Drawing for the job (mm, zero at the part's lowest x, y, z). A direction names the side the tool comes from. Give positions to 0.01 mm unless a question says otherwise; leave off trailing zeros. Write each loop counter-clockwise with the first axis right and the second up, starting at its lowest first coordinate (ties: lowest second). Pieces come first, ordered by that corner, then holes. Notation, with made-up numbers: M -1.5,3 L 40.5,3 A27 cw 40.5,25 Z; hole C -33,39.25 d6. An arc over 180 degrees is marked long. Use CSV: the item, a comma, the result in double quotes. Start each with the question number.
1. Band-saw the part on D-D, the plane z = 17. List the corners of the cut face in (x, y), then the cut area to 3 significant figures.
2. Band-saw the part on A-A, the plane x = 36.5. List the corners of the cut face in (y, z), then the cut area to 3 significant figures.
3. 3-axis set-ups, long thin cutter, end or side, ignore diameter. For the marked faces 1, 2, 3 and 4: which of +Z, -Z, +X, -X, +Y, -Y reach the whole face in a straight line?
4. Drop flat-ended pins along their axis: pin 1 Ø4.5 at (x, y) = (14, 8) entering from +Z; pin 2 Ø6 at (x, y) = (20.5, 43.5) entering from +Z; pin 3 Ø3 at (y, z) = (5, 30) entering from +X. Give the stop position or say it passes through.
5. Drill centre lines: line 1 along Y through (x, z) = (60, 21); line 2 along Z through (x, y) = (67, 20); line 3 along Y through (x, z) = (60, 26). Where is each one in solid material? Low to high. Write a range as from..to.
6. Mould opens along X. For the marked faces 5, 6 and 7 say: pulls with the +X half, pulls with the -X half, needs draft (parallel to the pull), parting line crosses it, or undercut.
7. Band-saw the part on B-B, the plane z = 8. List the corners of the cut face in (x, y).
8. Band-saw the part on C-C, the plane y = 53. List the corners of the cut face in (x, z).
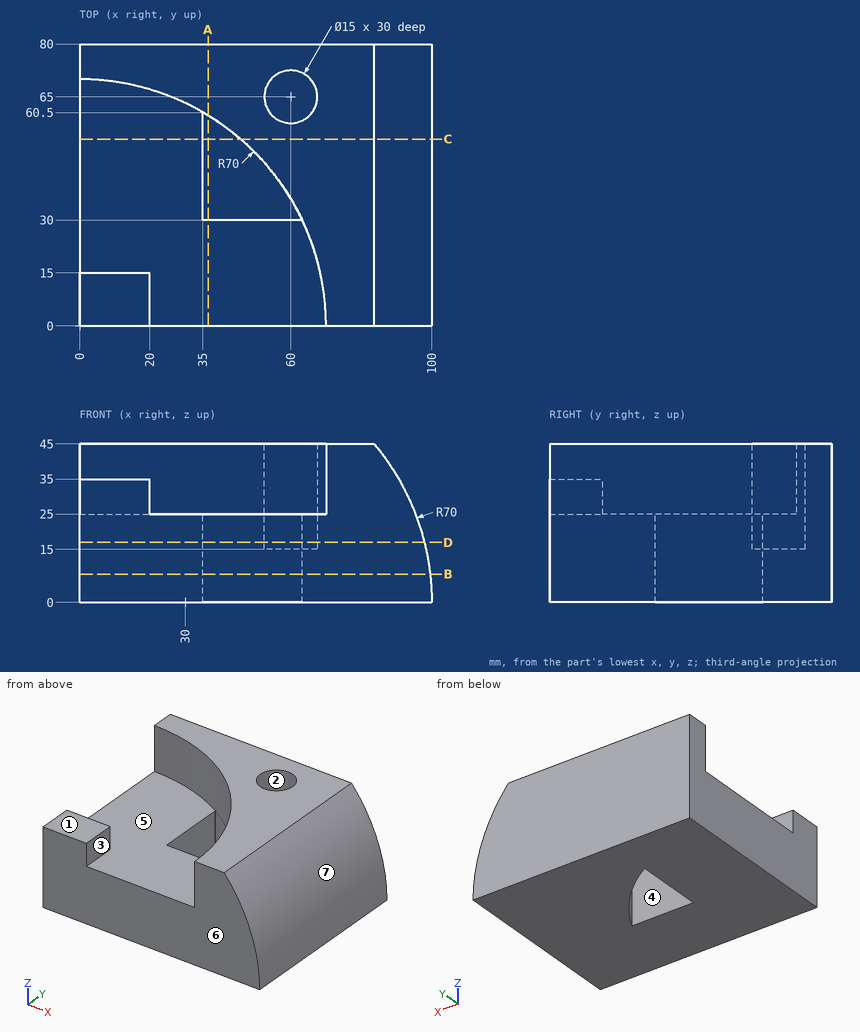
Output:
1,outline,"M 0,0 L 97.9,0 L 97.9,80 L 0,80 Z; hole M 35,30 L 63.25,30 A70 ccw 35.21,60.5 L 35,60.5 Z; hole C 60,65 d15"
1,area,"7,130 mm²"
2,outline,"M 0,0 L 30,0 L 30,25 L 0,25 Z; M 59.73,0 L 80,0 L 80,45 L 59.73,45 Z"
2,area,"1,660 mm²"
3,face 1,"+Z, -X, -Y"
3,face 2,"+Z"
3,face 3,"+Z, -Y"
3,face 4,"+Z, -Z"
4,pin 1,"stops at z = 35"
4,pin 2,"stops at z = 25"
4,pin 3,"stops at x = 93.94"
5,line 1,"y = 0..30, 36.06..57.5, 72.5..80"
5,line 2,"z = 0..25"
5,line 3,"y = 36.06..57.5, 72.5..80"
6,face 5,"undercut"
6,face 6,"needs draft"
6,face 7,"pulls with the +X half"
7,outline,"M 0,0 L 99.54,0 L 99.54,80 L 0,80 Z; hole M 35,30 L 63.25,30 A70 ccw 35.21,60.5 L 35,60.5 Z"
8,outline,"M 0,0 L 35,0 L 35,25 L 0,25 Z; M 45.73,0 L 100,0 A70 ccw 83.62,45 L 45.73,45 Z"
